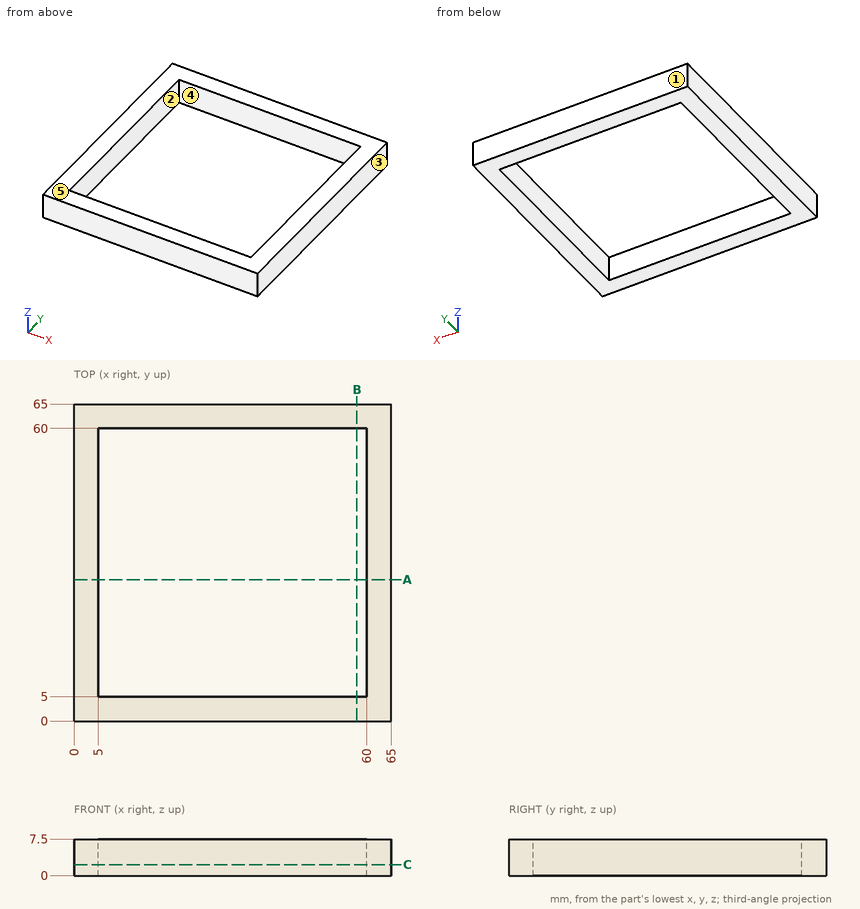
For this review, use the dimensioned drawing (mm, ordinates from the lowest corner) and the shaded views. A direction names the side the tool comes from. Coordinates: 2 decimals unless noted, no trailing zeros. Write each loop counter-clockwise with the first axis right and the second up, starting at its lowest first coordinate (ties: lowest second). Pieces come first, ordered by that corner, then holes. Notation, with made-up numbers: (51.5, -0.75) -> (82.5, -0.75) arc R21 ccw to (82.5, 11.25) -> close; hole circle Ø10 at (7, -12). An arc over 180 degrees is marked (long way). Put each result on its own line as item: value.
Q1. Take a section at C-C, the plane z = 2.25. State the section outline as (x, y) points, then the cut area to 3 significant figures.
From the geometry:
outline: (0, 0) -> (65, 0) -> (65, 65) -> (0, 65) -> close; hole (5, 5) -> (60, 5) -> (60, 60) -> (5, 60) -> close
area: 1,200 mm2
Q2. Tool access review of the marked faces 1 and 2: name each direction out of +Z, -Z, +X, -X, +Y, -Y from which nothing blocks a thin tool from reaching the whole face with its end or side.
From the geometry:
face 1: +Z, -Z, +X, -X, +Y
face 2: +Z, -Z
Q3. The part is to be moulded in two halves that separate along X. For the marked faces 3, 4 and 5, say which applies: +X half, -X half, draft (parallel to the pull), parting line (faces both ways), or undercut.
From the geometry:
face 3: +X half
face 4: undercut
face 5: draft
Q4. Clearance check with a flat-ended pin moving along its axis: pin 1 Ø4 at (y, z) = (44.5, 3) entering from -X. State where the tip first meets the part, or that it passes through.
From the geometry:
pin 1: stops at x = 0
Q5. Take a section at A-A, the plane y = 29. State the section outline as (x, z) points.
From the geometry:
outline: (0, 0) -> (5, 0) -> (5, 7.5) -> (0, 7.5) -> close; (60, 0) -> (65, 0) -> (65, 7.5) -> (60, 7.5) -> close
Q6. Wall thickness on L1, parallel to X at y = 30, z = 5: over which ranges is the line inside the solid? List them lowest first.
From the geometry:
L1: x = 0 to 5, 60 to 65
